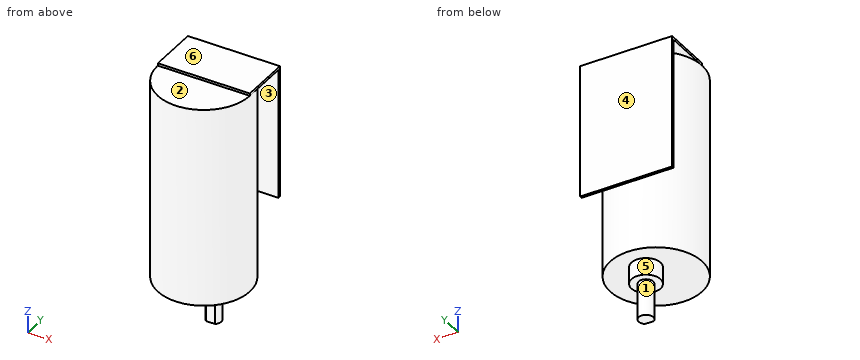
from build123d import *

# Parameters (mm, degrees)
SKETCH_R     = 19
PAD_DEPTH    = 82.6
SKETCH001_R  = 6
PAD001_DEPTH = 7
PAD002_DEPTH = 15
SKETCH003_W  = 38
SKETCH003_H  = 19.65
PAD003_DEPTH = 1
SKETCH005_W  = 38
SKETCH005_H  = 55
PAD004_DEPTH = 1


with BuildPart() as part:
    # Sketch → Pad (new body)
    with BuildSketch(Plane.XY):
        Circle(SKETCH_R)
    extrude(amount=PAD_DEPTH)

    # Sketch001 → Pad001 (new body)
    with BuildSketch(Plane(origin=(0, 0, 0), x_dir=(1, 0, 0), z_dir=(0, 0, -1))):
        with Locations((0, -7)):
            Circle(SKETCH001_R)
    extrude(amount=PAD001_DEPTH)

    # Sketch002 → Pad002 (new body)
    with BuildSketch(Plane(origin=(0, 0, -7), x_dir=(1, 0, 0), z_dir=(0, 0, -1))):
        with BuildLine():
            Line((-1.85, -4.638327), (1.85, -4.638327))
            ThreePointArc((-1.85, -4.638327), (0, -10), (1.85, -4.638327))
        make_face()
    extrude(amount=PAD002_DEPTH)

    # Sketch003 → Pad003 (new body)
    with BuildSketch(Plane.XY.offset(82.6)):
        with Locations((0, 9.825)):
            Rectangle(SKETCH003_W, SKETCH003_H)
    extrude(amount=PAD003_DEPTH)

    # Sketch005 → Pad004 (new body)
    with BuildSketch(Plane(origin=(0, 19.65, 0), x_dir=(-1, 0, 0), z_dir=(0, 1, 0))):
        with Locations((0, 56.1)):
            Rectangle(SKETCH005_W, SKETCH005_H)
    extrude(amount=PAD004_DEPTH)


solid = part.part
Verification items for the finished model (mm, model axes). Face numbers are marked on the shaded views. A direction names the side the tool comes from. Round coordinates to 2 decimals unless told otherwise and drop trailing zeros. Order: outer loops, then holes, each group sorted by start corner. A loop starts at its lowest first (then second) coordinate and runs counter-clockwise, first axis right, second up.
1. Section check D-D on z = 15. Record the cut outline in (x, y), then the cut area to 3 significant figures.
Final values:
outline: circle Ø38 at (0, 0)
area: 1,130 mm2
2. Section check B-B on x = 0. Record the cut outline in (y, z), then the cut area to 3 significant figures.
Final values:
outline: (-19, 0) - (1, 0) - (1, -7) - (4.64, -7) - (4.64, -22) - (10, -22) - (10, -7) - (13, -7) - (13, 0) - (19, 0) - (19, 82.6) - (19.65, 82.6) - (19.65, 28.6) - (20.65, 28.6) - (20.65, 83.6) - (0, 83.6) - (0, 82.6) - (-19, 82.6) - close
area: 3,380 mm2
3. Section check C-C on y = 16. Record the cut outline in (x, z).
Final values:
outline: (-19, 82.6) - (-10.25, 82.6) - (-10.25, 0) - (10.25, 0) - (10.25, 82.6) - (19, 82.6) - (19, 83.6) - (-19, 83.6) - close
4. Thickness scan on L1, parallel to Z at x = 13, y = 7.5; L2, parallel to Z at x = 2.5, y = -13.5; L3, parallel to Y at x = -1.5, z = 33.5. Record the ranges inside material, lowest first.
Final values:
L1: z = 0 to 83.6
L2: z = 0 to 82.6
L3: y = -18.94 to 18.94, 19.65 to 20.65
5. Section check A-A on z = 43. Record the cut outline in (x, y).
Final values:
outline: circle Ø38 at (0, 0); (-19, 19.65) - (19, 19.65) - (19, 20.65) - (-19, 20.65) - close
6. Release check for a two-part mould opening along Y. For the marked faces 1, 2, 3 and 4 record: +Y half, -Y half, draft (parallel to the pull), parting line (faces both ways), or undercut.
Final values:
face 1: parting line
face 2: draft
face 3: undercut
face 4: +Y half
7. Access from +Z, -Z, +X, -X, +Y, -Y to the whole of each face (thin tool, end or side, straight path). Record for the marked faces 5 and 6.
Final values:
face 5: -Z
face 6: +Z, +X, -X, +Y, -Y
8. Go/stop test with flat-tipped pins: P1, Ø6, axis at y = 15, z = 41.5, coming from the -X side; P2, Ø0.8, axis at x = 6, y = 20.5, coming from the -Z side; P3, Ø1.5, axis at x = 6.5, y = -15, coming from the +Z side. Record where each tip stops, or that it passes through.
Final values:
P1: stops at x = -14.73
P2: stops at z = 28.6
P3: stops at z = 82.6
